Here's the drawing with two shaded views (mm, measured from the low corner). I have some questions. A direction names the side the tool comes from. Round coordinates to 2 decimals unless told otherwise and drop trailing zeros. Loops run counter-clockwise (first coordinate to the right, second up) from the corner with the lowest first, then second, coordinate; pieces in that order, holes last. Notation, with made-up numbers: (7.5, 8) - (51.5, 8) arc R21 cw to (51.5, 19) - close; hole circle Ø11 at (81, -9). An arc over 180 degrees is marked (long way). Use one line per item in the form item = value.
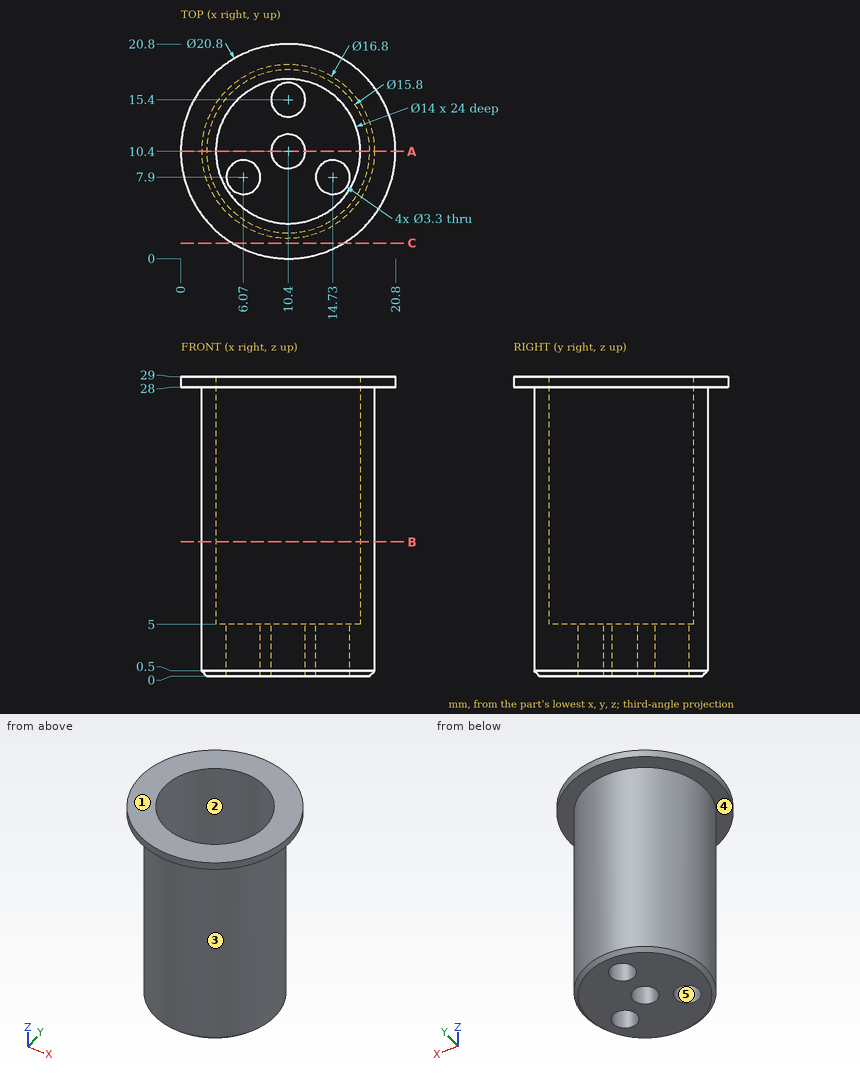
1. If we section it at C-C, the plane y = 1.5: Write out the boundary of the cut face in (x, z).
Solution:
outline = (5.02, 28) - (15.78, 28) - (15.78, 29) - (5.02, 29) - close
2. Please list where these lines run through material, in increasing order: line 1 along Y through (x, z) = (10.4, 1.5); line 2 along Y through (x, z) = (10.4, 11); line 3 along Y through (x, z) = (9, 27.75).
Solution:
line_1 = 2 to 8.75, 12.05 to 13.75, 17.05 to 18.8
line_2 = 2 to 3.4, 17.4 to 18.8
line_3 = 2.12 to 3.54, 17.26 to 18.68
3. If we section it at B-B, the plane z = 13: Write out the boundary of the cut face in (x, y).
Solution:
outline = circle Ø16.8 at (10.4, 10.4); hole circle Ø14 at (10.4, 10.4)
4. If we section it at A-A, the plane y = 10.4: Write out the boundary of the cut face in (x, z), plus the area to 3 significant figures.
Solution:
outline = (0, 28) - (2, 28) - (2, 0.5) - (2.5, 0) - (8.75, 0) - (8.75, 5) - (3.4, 5) - (3.4, 29) - (0, 29) - close; (12.05, 0) - (18.3, 0) - (18.8, 0.5) - (18.8, 28) - (20.8, 28) - (20.8, 29) - (17.4, 29) - (17.4, 5) - (12.05, 5) - close
area = 138 mm^2
5. For P1, Ø8.5, axis at x = 10.4, y = 10.4, coming from the +Z side; P2, Ø4, axis at y = 2, z = 21, coming from the +X side; P3, Ø4, axis at x = 13.5, z = 21.5, coming from the +Y side, each with a flat end and sliding along its axis, tell me the tip position at first contact or that it passes through.
Solution:
P1 = 5
P2 = 15.84
P3 = 18.73
6. We'd pull the mould along X, two halves only. Please class the marked faces 3, 4 and 5: +X half, -X half, draft (parallel to the pull), parting line (faces both ways), or undercut.
Solution:
face_3 = parting line
face_4 = draft
face_5 = undercut
7. On a 3-axis mill with a long thin cutter (end or side, diameter ignored), from which of +Z, -Z, +X, -X, +Y, -Y can I reach the whole of each face in a straight line? I mean the marked faces 1 and 2. Say none if no direction works.
Solution:
face_1 = +Z, +X, -X, +Y, -Y
face_2 = +Z
